Check sheet for the drawn part. Datum: minimum x, y, z corner. Units: mm. A direction names the side the tool comes from. Give positions to 0.01 mm unless a question says otherwise; leave off trailing zeros. Order: outer loops, then holes, each group sorted by start corner. A loop starts at its lowest first (then second) coordinate and runs counter-clockwise, first axis right, second up. Notation, with made-up numbers: (1, 81) -> (8, 81) arc R16 ccw to (8, 106) -> close; hole circle Ø5 at (-18, 66). An arc over 180 degrees is marked (long way). Return JSON: item names as keys, results as strings. Group by question number.
(1) Release check for a two-part mould opening along X. For the marked faces 3 and 4 record: pulls with the +X half, pulls with the -X half, needs draft (parallel to the pull), parting line crosses it, or undercut.
(2) Depth check by flat-ended pin: pin 1 Ø12 at (x, y) = (3.5, 14) entering from +Z; pin 2 Ø6 at (x, y) = (7.5, 14) entering from +Z. Enter the tip coordinate at first touch or a pass-through.
(3) Cross-section at A-A on y = 13. Enter the section's corners in (x, z).
(4) Thickness scan on line 1 along X through (y, z) = (13, 2.3); line 2 along Y through (x, z) = (13, 1.5). Record the ranges inside material, lowest first.
(5) Cross-section at C-C on z = 2.4. Enter the section's corners in (x, y).
(6) Tool access check on the marked faces 1 and 2. Record the directions out of +Z, -Z, +X, -X, +Y, -Y that give a thin tool (end or side, any length) a straight path to the whole face; none if there is none.
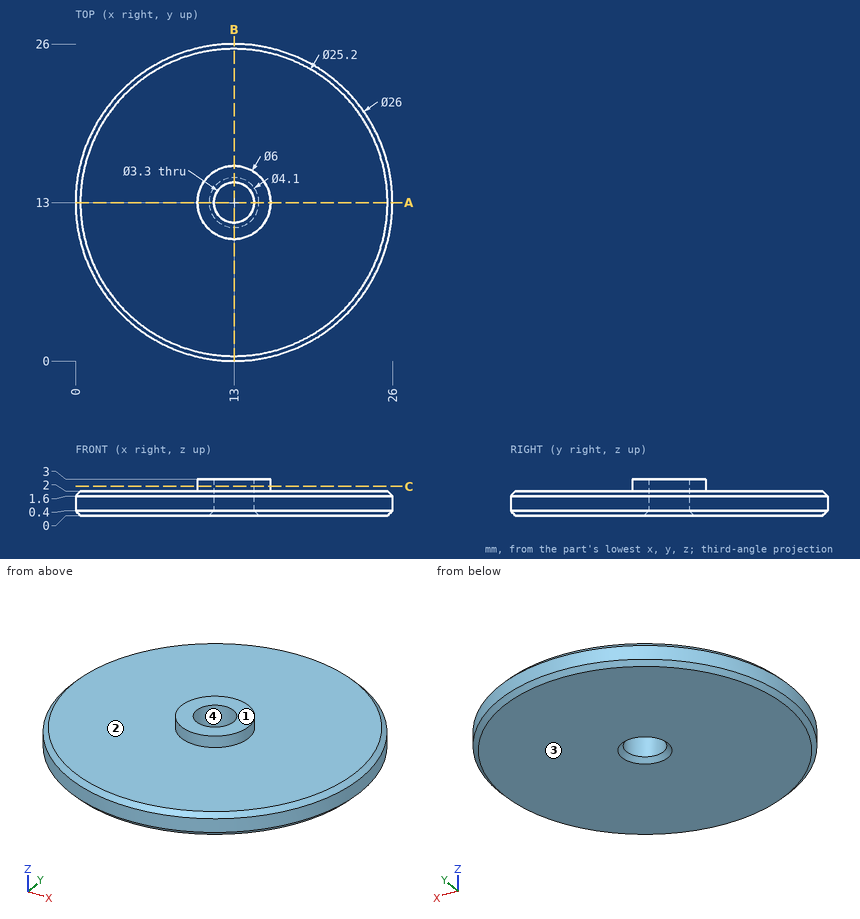
Verdict:
{
 "1": {"face 3": "needs draft", "face 4": "undercut"},
 "2": {"pin 1": "z = 2", "pin 2": "z = 3"},
 "3": {"outline": "(0, 0.4) -> (0.4, 0) -> (10.95, 0) -> (11.35, 0.4) -> (11.35, 3) -> (10, 3) -> (10, 2) -> (0.4, 2) -> (0, 1.6) -> close; (14.65, 0.4) -> (15.05, 0) -> (25.6, 0) -> (26, 0.4) -> (26, 1.6) -> (25.6, 2) -> (16, 2) -> (16, 3) -> (14.65, 3) -> close"},
 "4": {"line 1": "10 to 11.35, 14.65 to 16", "line 2": "0 to 11.35, 14.65 to 26"},
 "5": {"outline": "circle Ø6 at (13, 13); hole circle Ø3.3 at (13, 13)"},
 "6": {"face 1": "+Z, +X, -X, +Y, -Y", "face 2": "+Z"}
}
